```python
from build123d import *

# Parameters (mm, degrees)
SKETCH1_W           = 40
SKETCH1_H           = 200
BOSS_EXTRUDE1_DEPTH = 20
SKETCH2_R           = 2.125
BOSS_EXTRUDE2_DEPTH = 5
BOSS_EXTRUDE3_START = 5
SKETCH3_R           = 2.125
BOSS_EXTRUDE3_DEPTH = 5
SKETCH4_W           = 35
SKETCH4_H           = 35
CUT_EXTRUDE1_DEPTH  = 210.5
CUT_EXTRUDE2_DEPTH  = 210.5
CUT_EXTRUDE3_DEPTH  = 210.5
BOSS_EXTRUDE4_DEPTH = 40
SKETCH8_W           = 35
SKETCH8_H           = 4.25
CUT_EXTRUDE4_DEPTH  = 141
CUT_EXTRUDE5_DEPTH  = 50
BOSS_EXTRUDE5_DEPTH = 40
SKETCH16_W          = 35
SKETCH16_H          = 4.25
CUT_EXTRUDE6_DEPTH  = 40
SKETCH17_W          = 6.375
SKETCH17_H          = 17.5
CUT_EXTRUDE7_DEPTH  = 53
BOSS_EXTRUDE6_DEPTH = 6.375


with BuildPart() as part:
    # Sketch1 → Boss-Extrude1 (new body)
    with BuildSketch(Plane(origin=(0, 0, 0), x_dir=(1, 0, 0), z_dir=(0, 1, 0))):
        Rectangle(SKETCH1_W, SKETCH1_H)
    extrude(amount=BOSS_EXTRUDE1_DEPTH)

    # Sketch2 → Boss-Extrude2 (add)
    with BuildSketch(Plane(origin=(20, 0, 0), x_dir=(0, 0, -1), z_dir=(1, 0, 0))):
        with Locations(Location((-95.75, 4.125, 0), (0, 0, 180))):
            Circle(SKETCH2_R)
    extrude(amount=BOSS_EXTRUDE2_DEPTH)

    # Sketch3 → Boss-Extrude3 (add)
    with BuildSketch(Plane.ZY.offset(20).offset(BOSS_EXTRUDE3_START)):
        with Locations((95.75, 4.125)):
            Circle(SKETCH3_R)
    extrude(amount=-BOSS_EXTRUDE3_DEPTH)

    # Sketch4 → Cut-Extrude1 (cut)
    with BuildSketch(Plane.XY.offset(100)):
        with Locations((0, 20)):
            Rectangle(SKETCH4_W, SKETCH4_H)
    extrude(amount=-CUT_EXTRUDE1_DEPTH, mode=Mode.SUBTRACT)

    # Sketch5 → Cut-Extrude2 (cut)
    with BuildSketch(Plane.ZY.offset(20)):
        Polygon((-100, 0), (-95, 0), (-95, 17.5), (100, 17.5), (100, 20), (-100, 20), align=None)
    extrude(amount=-CUT_EXTRUDE2_DEPTH, mode=Mode.SUBTRACT)

    # Sketch6 → Cut-Extrude3 (cut)
    with BuildSketch(Plane.ZY.offset(20)):
        with BuildLine():
            Line((-90.75, 15.5), (95.75, 15.5))
            ThreePointArc((95.75, 15.5), (97.875, 13.375), (95.75, 11.25))
            Line((95.75, 11.25), (-90.75, 11.25))
            ThreePointArc((-90.75, 11.25), (-92.875, 13.375), (-90.75, 15.5))
        make_face()
    extrude(amount=-CUT_EXTRUDE3_DEPTH, mode=Mode.SUBTRACT)

    # Sketch7 → Boss-Extrude4 (add)
    with BuildSketch(Plane.ZY.offset(20)):
        with BuildLine():
            Line((6.75, 11.25), (-95, 11.25))
            Line((-95, 11.25), (-95, 15.5))
            Line((-95, 15.5), (6.75, 15.5))
            ThreePointArc((6.75, 15.5), (4.625, 13.375), (6.75, 11.25))
        make_face()
    extrude(amount=-BOSS_EXTRUDE4_DEPTH)

    # Sketch8 → Cut-Extrude4 (cut)
    with BuildSketch(Plane(origin=(0, 0, -95), x_dir=(-1, 0, 0), z_dir=(0, 0, -1))):
        with Locations((0, 13.375)):
            Rectangle(SKETCH8_W, SKETCH8_H)
    extrude(amount=-CUT_EXTRUDE4_DEPTH, mode=Mode.SUBTRACT)

    # Sketch14 → Cut-Extrude5 (cut)
    with BuildSketch(Plane.ZY.offset(20)):
        with BuildLine():
            Line((0.375, 11.25), (6.75, 11.25))
            Line((6.75, 11.25), (6.75, 15.5))
            Line((6.75, 15.5), (0.375, 15.5))
            ThreePointArc((0.375, 15.5), (-1.75, 13.375), (0.375, 11.25))
        make_face()
    extrude(amount=-CUT_EXTRUDE5_DEPTH, mode=Mode.SUBTRACT)

    # Sketch15 → Boss-Extrude5 (add)
    with BuildSketch(Plane.ZY.offset(20)):
        with BuildLine():
            Line((95.75, 15.5), (91.5, 15.5))
            ThreePointArc((91.5, 15.5), (93.625, 13.375), (91.5, 11.25))
            Line((91.5, 11.25), (95.75, 11.25))
            ThreePointArc((95.75, 11.25), (97.875, 13.375), (95.75, 15.5))
        make_face()
    extrude(amount=-BOSS_EXTRUDE5_DEPTH)

    # Sketch16 → Cut-Extrude6 (cut)
    with BuildSketch(Plane.XY.offset(100)):
        with Locations((0, 13.375)):
            Rectangle(SKETCH16_W, SKETCH16_H)
    extrude(amount=-CUT_EXTRUDE6_DEPTH, mode=Mode.SUBTRACT)

    # Sketch17 → Cut-Extrude7 (cut)
    with BuildSketch(Plane.ZY.offset(20)):
        with Locations((-91.8125, 8.75)):
            Rectangle(SKETCH17_W, SKETCH17_H)
    extrude(amount=-CUT_EXTRUDE7_DEPTH, mode=Mode.SUBTRACT)

    # Sketch18 → Boss-Extrude6 (add)
    with BuildSketch(Plane.XY.offset(100)):
        Polygon((-20, 17.5), (-17.5, 17.5), (-17.5, 2.5), (17.5, 2.5), (17.5, 17.5), (20, 17.5), (20, 0), (-20, 0), align=None)
    extrude(amount=BOSS_EXTRUDE6_DEPTH)


solid = part.part
```
Model file for the job. Use its own axes, mm. A direction names the side the tool comes from. Give positions to 0.01 mm unless a question says otherwise; leave off trailing zeros. Loops run counter-clockwise (first coordinate to the right, second up) from the corner with the lowest first, then second, coordinate; pieces in that order, holes last. Notation, with made-up numbers: M -29,72.25 L 14,72.25 A20 cw 14,106.25 Z; hole C -38.75,55 d5. An arc over 180 degrees is marked long. Use one line per item in the form item = value.
Item 1: Which spindle directions (+Z, -Z, +X, -X, +Y, -Y) get a long thin tool onto all of the face, cutting with end or side? Do faces 4 (the cylindrical face through (-22.535, 2.832, 94.064)), 5 (the flat face through (1, 2, -88.625)), 6 (the flat face through (-17.5, 10, 8)), 7 (the cylindrical face through (22.465, 5.418, 94.064)). Say none if no direction does.
Filled in:
face_4 = -X
face_5 = -Z, +X, -X, +Y, -Y
face_6 = +Z, -Z, +Y
face_7 = +X
Item 2: Drill centre lines: L1, parallel to X at y = 7, z = -28.5; L2, parallel to Y at x = -1, z = -40; L3, parallel to X at y = 2, z = -61. Where is each one in solid material? Low to high.
Filled in:
L1 = -20 to -17.5, 17.5 to 20
L2 = 0 to 2.5
L3 = -20 to 20
Item 3: Slice it at A-A on z = 87. List the corners of the cut face in (x, y).
Filled in:
outline = M -20,0 L 20,0 L 20,11.25 L 17.5,11.25 L 17.5,2.5 L -17.5,2.5 L -17.5,11.25 L -20,11.25 Z; M -20,15.5 L -17.5,15.5 L -17.5,17.5 L -20,17.5 Z; M 17.5,15.5 L 20,15.5 L 20,17.5 L 17.5,17.5 Z
Item 4: Two-plate mould, pull along X, no slides. Class faces 1 (the flat face through (17.5, 10, 8)), 2 (the flat face through (-20, 9, 8)), 3 (the flat face through (25, 4, 96)): released by +X, released by -X, zero draft, split by the parting line, or undercut.
Filled in:
face_1 = undercut
face_2 = released by -X
face_3 = released by +X
Item 5: Slice it at C-C on z = -50. List the corners of the cut face in (x, y).
Filled in:
outline = M -20,0 L 20,0 L 20,17.5 L 17.5,17.5 L 17.5,2.5 L -17.5,2.5 L -17.5,17.5 L -20,17.5 Z
Item 6: Slice it at D-D on x = -10. List the corners of the cut face in (y, z) (3 decimals).
Filled in:
outline = M 0,-88.625 L 2.5,-88.625 L 2.5,106.375 L 0,106.375 Z
Item 7: Flat gauge pins, fed straight in: pin 1 Ø10 at (y, z) = (3.5, -16) entering from -X; pin 2 Ø4.5 at (y, z) = (6.5, 17) entering from +X; pin 3 Ø17.5 at (x, z) = (-6, -5.5) entering from +Y. Where does each tip first touch, or does it go through?
Filled in:
pin_1 = -20
pin_2 = 20
pin_3 = 2.5
Item 8: Slice it at B-B on y = 13. List the corners of the cut face in (x, z) (3 decimals).
Filled in:
outline = M -20,-88.625 L -17.5,-88.625 L -17.5,-1.717 L -20,-1.717 Z; M -20,93.592 L -17.5,93.592 L -17.5,106.375 L -20,106.375 Z; M 17.5,-88.625 L 20,-88.625 L 20,-1.717 L 17.5,-1.717 Z; M 17.5,93.592 L 20,93.592 L 20,106.375 L 17.5,106.375 Z
